Could you check a few things on this model? Use its own coordinates, in mm. Coordinates: 2 decimals unless noted, no trailing zeros. Loops run counter-clockwise (first coordinate to the right, second up) from the corner with the lowest first, then second, coordinate; pieces in that order, holes last. Notation, with made-up numbers: M -21,-28.75 L 19,-28.75 A23 cw 19,-6.75 Z; hole C 18,-36.5 d8. An arc over 180 degrees is marked long. Write each question's results on one line, items separated by ' | '.
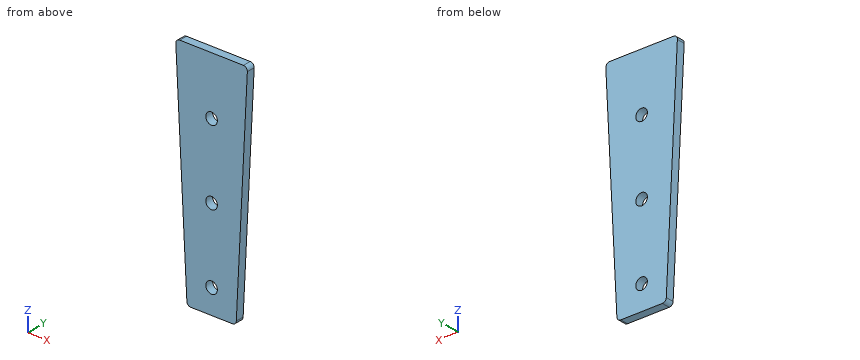
```python
from build123d import *

# Parameters (mm, degrees)
BOSS_EXTRUDE1_DEPTH  = 3.175
M4_CLEARANCE_HOLE1_D = 4.5


with BuildPart() as part:
    # Sketch1 → Boss-Extrude1 (new body)
    with BuildSketch(Plane(origin=(0, 0, 0), x_dir=(1, 0, 0), z_dir=(0, 1, 0))):
        with BuildLine():
            Line((-75.32, 38.035000003), (-67.244703811, 38.035000003))
            ThreePointArc((-67.244703811, 38.035000003), (-66.19432481, 37.615210108), (-65.722605246, 36.587104931))
            Line((-65.722605246, 36.587104931), (-61.430005246, -49.264895069))
            ThreePointArc((-61.430005246, -49.264895069), (-61.847893706, -50.391378998), (-62.952103811, -50.864999997))
            Line((-62.952103811, -50.864999997), (-75.32, -50.864999997))
            Line((-75.32, -50.864999997), (-87.687896189, -50.864999997))
            ThreePointArc((-87.687896189, -50.864999997), (-88.792106294, -50.391378998), (-89.209994754, -49.264895069))
            Line((-89.209994754, -49.264895069), (-84.917394754, 36.587104931))
            ThreePointArc((-84.917394754, 36.587104931), (-84.44567519, 37.615210108), (-83.395296189, 38.035000003))
            Line((-83.395296189, 38.035000003), (-75.32, 38.035000003))
        make_face()
    extrude(amount=BOSS_EXTRUDE1_DEPTH)

    # M4 Clearance Hole1 (through all)
    with Locations(Plane(origin=(0, 3.175, 0), x_dir=(1, 0, 0), z_dir=(0, 1, 0))):
        with Locations((-75.32, 28.575), (-75.32, 0), (-75.32, -28.575)):
            Hole(M4_CLEARANCE_HOLE1_D / 2)


solid = part.part
```
(1) Imagine slicing it at B-B, the plane x = -75.32. List the corners of the cut face in (y, z) for me (3 decimals), and give its area (3 significant figures).
Reported:
outline: M 0,-38.035 L 3.175,-38.035 L 3.175,-30.825 L 0,-30.825 Z; M 0,-26.325 L 3.175,-26.325 L 3.175,-2.25 L 0,-2.25 Z; M 0,2.25 L 3.175,2.25 L 3.175,26.325 L 0,26.325 Z; M 0,30.825 L 3.175,30.825 L 3.175,50.865 L 0,50.865 Z | area: 239 mm2
(2) Imagine slicing it at D-D, the plane z = 34. List the corners of the cut face in (x, y) for me (3 decimals), and give its area (3 significant figures).
Reported:
outline: M -88.447,0 L -62.193,0 L -62.193,3.175 L -88.447,3.175 Z | area: 83.4 mm2
(3) Will this pin go through, and if not, where does the flat tip stop? P1, Ø4, axis at x = -75.32, z = -28.575, coming from the -Y side.
Reported:
P1: passes through
(4) Please list where these lines run through material, in increasing order: probe 1 along Z at (x, y) = (-75.32, 1.7) (3 decimals); probe 2 along Z at (x, y) = (-76.25, 2.95) (3 decimals); probe 3 along X at (y, z) = (2.35, -30.5). Write a range as from..to.
Reported:
probe 1: z = -38.035..-30.825, -26.325..-2.25, 2.25..26.325, 30.825..50.865 | probe 2: z = -38.035..-30.624, -26.526..-2.049, 2.049..26.526, 30.624..50.865 | probe 3: x = -85.22..-76.48, -74.16..-65.42
(5) Imagine slicing it at C-C, the plane y = 0.95. List the corners of the cut face in (x, z) for me (3 decimals).
Reported:
outline: M -89.21,49.265 L -84.917,-36.587 A1.524 ccw -83.395,-38.035 L -67.245,-38.035 A1.524 ccw -65.723,-36.587 L -61.43,49.265 A1.524 ccw -62.952,50.865 L -87.688,50.865 A1.524 ccw Z; hole C -75.32,-28.575 d4.5; hole C -75.32,0 d4.5; hole C -75.32,28.575 d4.5
(6) Imagine slicing it at A-A, the plane z = 0. List the corners of the cut face in (x, y) for me (3 decimals), and give its area (3 significant figures).
Reported:
outline: M -86.747,0 L -77.57,0 L -77.57,3.175 L -86.747,3.175 Z; M -73.07,0 L -63.893,0 L -63.893,3.175 L -73.07,3.175 Z | area: 58.3 mm2
